The model under review builds one solid part; all positions refer to its coordinate system, in mm. A direction names the side the tool comes from. Coordinates: 2 decimals unless noted, no trailing zeros. Loops run counter-clockwise (first coordinate to the right, second up) from the corner with the lowest first, then second, coordinate; pieces in that order, holes last. Notation, with made-up numbers: (69, -24.5) - (119, -24.5) arc R14 ccw to (119, -11.5) - close; hole circle Ø1 at (-10, -25.75). An arc over 180 degrees is marked (long way). One line per item, written item: value. Start each with the question number.
1. We need section A-A, the plane z = 2. Give the boundary of the cut face in (x, y).
2. To check wall thickness, follow line 1 (Z direction, x = 10, y = 7.25); line 2 (X direction, y = 2, z = 7.25); line 3 (Y direction, x = -2.5, z = 8). State the ranges of each line that lie inside material, in increasing order.
3. We need section B-B, the plane y = 0. Give the boundary of the cut face in (x, z).
4. For faces 4 (the face through (6, -6, 3)), 5 (the face through (10.69, -5.18, 1.48)), list the 3-axis set-ups (+Z, -Z, +X, -X, +Y, -Y) from which the entire face can be reached by the end or side of a thin tool; tool diameter is ignored.
5. Insertion check: P1, Ø5, axis at x = -9.09, y = -5.25, coming from the +Z side; P2, Ø2, axis at y = 4.5, z = 2.5, coming from the +X side; P3, Ø1, axis at y = 0, z = 8.5, coming from the -X side. Each pin has a flat end and moves straight along its axis. Give the tip position at first contact, or say it passes through.
6. We need section D-D, the plane y = -5.25. Give the boundary of the cut face in (x, z), then the cut area to 3 significant figures.
7. We need section C-C, the plane x = -7. Give the boundary of the cut face in (y, z).
8. Mouldability with a two-part tool opening along X and no side actions: class faces 1 (the face through (-7.495, -5.18, 1.479)), 2 (the face through (-7.493, 0.33, 8.916)), 3 (the face through (-0.2, 3.3, 0)) as +X half, -X half, draft (parallel to the pull), parting line (faces both ways), or undercut.
from build123d import *

# Parameters (mm, degrees)
SKETCH_1_R          = 14
EXTRUDE_1_DEPTH     = 3
SKETCH_2_R          = 7.5
SKETCH_2_R_2        = 3
EXTRUDE_2_DEPTH     = 12
SKETCH_3_R          = 3
CUT_EXTRUDE_1_DEPTH = 4
SKETCH_4_R          = 1.6
CUT_EXTRUDE_2_DEPTH = 16


with BuildPart() as part:
    # 草图1 → 凸台-拉伸1 (new body)
    with BuildSketch(Plane.XY):
        Circle(SKETCH_1_R)
    extrude(amount=EXTRUDE_1_DEPTH)

    # 草图2 → 凸台-拉伸2 (add)
    with BuildSketch(Plane.XY.offset(3)):
        Circle(SKETCH_2_R)
        Circle(SKETCH_2_R_2, mode=Mode.SUBTRACT)
    extrude(amount=EXTRUDE_2_DEPTH)

    # 草图3 → 切除-拉伸1 (cut, through all)
    with BuildSketch(Plane.XY.offset(3)):
        Circle(SKETCH_3_R)
    extrude(amount=-CUT_EXTRUDE_1_DEPTH, mode=Mode.SUBTRACT)

    # 草图4 → 切除-拉伸2 (cut, through all)
    with BuildSketch(Plane(origin=(0, 0, 0), x_dir=(-1, 0, 0), z_dir=(0, 0, -1))):
        with Locations((-9.09326674, -5.25)):
            Circle(SKETCH_4_R)
        with Locations((9.09326674, 5.25)):
            Circle(SKETCH_4_R)
        with Locations((0, -10.5)):
            Circle(SKETCH_4_R)
        with Locations((9.09326674, -5.25)):
            Circle(SKETCH_4_R)
        with Locations((0, 10.5)):
            Circle(SKETCH_4_R)
        with Locations((-9.09326674, 5.25)):
            Circle(SKETCH_4_R)
    extrude(amount=-CUT_EXTRUDE_2_DEPTH, mode=Mode.SUBTRACT)


solid = part.part
Findings below:
1. outline: circle Ø28 at (0, 0); hole circle Ø3.2 at (-9.09, -5.25); hole circle Ø3.2 at (-9.09, 5.25); hole circle Ø6 at (0, 0); hole circle Ø3.2 at (0, -10.5); hole circle Ø3.2 at (0, 10.5); hole circle Ø3.2 at (9.09, -5.25); hole circle Ø3.2 at (9.09, 5.25)
2. line 1: 0 to 3
2. line 2: -7.23 to -2.24, 2.24 to 7.23
2. line 3: -7.07 to -1.66, 1.66 to 7.07
3. outline: (-14, 0) - (-3, 0) - (-3, 15) - (-7.5, 15) - (-7.5, 3) - (-14, 3) - close; (3, 0) - (14, 0) - (14, 3) - (7.5, 3) - (7.5, 15) - (3, 15) - close
4. face 4: +Z
4. face 5: +Z, -Z
5. P1: z = 3
5. P2: x = 13.56
5. P3: x = -7.5
6. outline: (-12.98, 0) - (-10.69, 0) - (-10.69, 3) - (-12.98, 3) - close; (-7.49, 0) - (7.49, 0) - (7.49, 3) - (5.36, 3) - (5.36, 15) - (-5.36, 15) - (-5.36, 3) - (-7.49, 3) - close; (10.69, 0) - (12.98, 0) - (12.98, 3) - (10.69, 3) - close
6. area: 187 mm2
7. outline: (-12.12, 0) - (12.12, 0) - (12.12, 3) - (2.69, 3) - (2.69, 15) - (-2.69, 15) - (-2.69, 3) - (-12.12, 3) - close
8. face 1: undercut
8. face 2: parting line
8. face 3: draft
